Input: dimensioned drawing with shaded views. Units: mm. Origin: part minimum x, y, z. A direction names the side the tool comes from. Coordinates: 2 decimals unless noted, no trailing zeros. Order: outer loops, then holes, each group sorted by start corner. A loop starts at its lowest first (then second) coordinate and runs counter-clockwise, first axis right, second up. Notation, with made-up numbers: (61, 71) -> (116, 71) arc R21 cw to (116, 87) -> close; hole circle Ø10 at (67.5, 11). An arc over 180 degrees is marked (long way). Put each result on its own line as item: value.
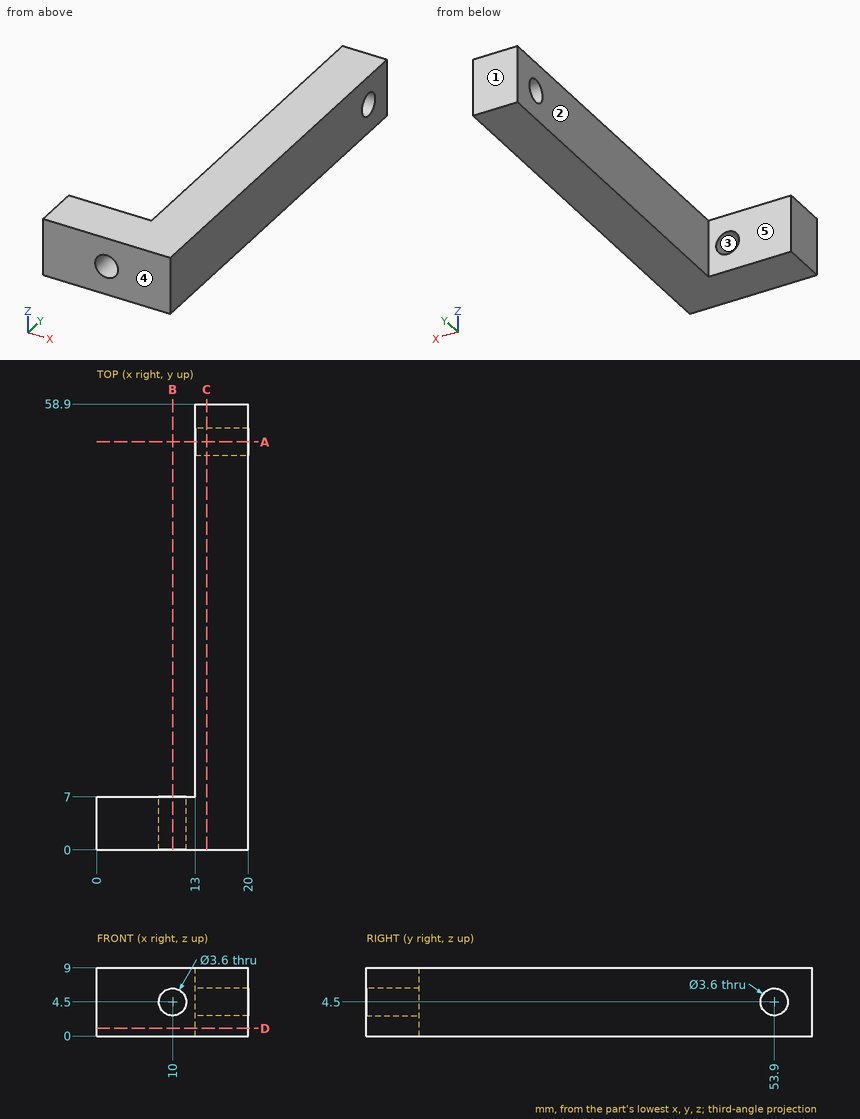
1. Set-up query: the marked faces 4 and 5. Return all of +Z, -Z, +X, -X, +Y, -Y with unobstructed straight access to the full face (end or side cutting, diameter ignored); none if empty.
Numbers:
face 4: +Z, -Z, +X, -X, -Y
face 5: +Z, -Z, -X, +Y
2. Cut plane A-A on y = 53.9. Output: boundary loops of the cut face in (x, z).
Numbers:
outline: (13, 0) -> (20, 0) -> (20, 2.7) -> (13, 2.7) -> close; (13, 6.3) -> (20, 6.3) -> (20, 9) -> (13, 9) -> close
3. Cut plane D-D on z = 1. Output: boundary loops of the cut face in (x, y), plus the area to 3 significant figures.
Numbers:
outline: (0, 0) -> (20, 0) -> (20, 58.9) -> (13, 58.9) -> (13, 7) -> (0, 7) -> close
area: 503 mm2
4. Cut plane B-B on x = 10. Output: boundary loops of the cut face in (y, z).
Numbers:
outline: (0, 0) -> (7, 0) -> (7, 2.7) -> (0, 2.7) -> close; (0, 6.3) -> (7, 6.3) -> (7, 9) -> (0, 9) -> close
5. Pull-direction query (X, two-part tool) for the marked faces 1, 2 and 3; classes: pulls with the +X half, pulls with the -X half, needs draft (parallel to the pull), parting line crosses it, or undercut.
Numbers:
face 1: needs draft
face 2: pulls with the -X half
face 3: undercut
6. Ray query, line 1 along X through (y, z) = (2.75, 4.5); line 2 along X through (y, z) = (10.5, 3.25); line 3 along Z through (x, y) = (17.5, 53.9). Return the intervals inside material, ascending.
Numbers:
line 1: x = 0 to 8.2, 11.8 to 20
line 2: x = 13 to 20
line 3: z = 0 to 2.7, 6.3 to 9
7. First-contact query: pin 1 (2.5 mm diameter, centred on x = 7, z = 5.5, fed in from +Y); pin 2 (1 mm diameter, centred on y = 28, z = 4.5, fed in from -X); pin 3 (3 mm diameter, centred on x = 10, z = 4.5, fed in from -Y). Flat tips, straight axial feed; report the tip coordinate or a pass-through.
Numbers:
pin 1: stops at y = 7
pin 2: stops at x = 13
pin 3: passes through
8. Cut plane C-C on x = 14.5. Output: boundary loops of the cut face in (y, z), plus the area to 3 significant figures.
Numbers:
outline: (0, 0) -> (58.9, 0) -> (58.9, 9) -> (0, 9) -> close; hole circle Ø3.6 at (53.9, 4.5)
area: 520 mm2
